For this review, use the dimensioned drawing (mm, ordinates from the lowest corner) and the shaded views. A direction names the side the tool comes from. Coordinates: 2 decimals unless noted, no trailing zeros. Order: outer loops, then holes, each group sorted by start corner. A loop starts at its lowest first (then second) coordinate and runs counter-clockwise, first axis right, second up. Notation, with made-up numbers: M -20.5,41 L 24.5,41 A25 ccw 24.5,69 Z; hole C 51.5,34 d4. An arc over 180 degrees is marked long. Use CSV: the item, a comma, the result in double quotes.
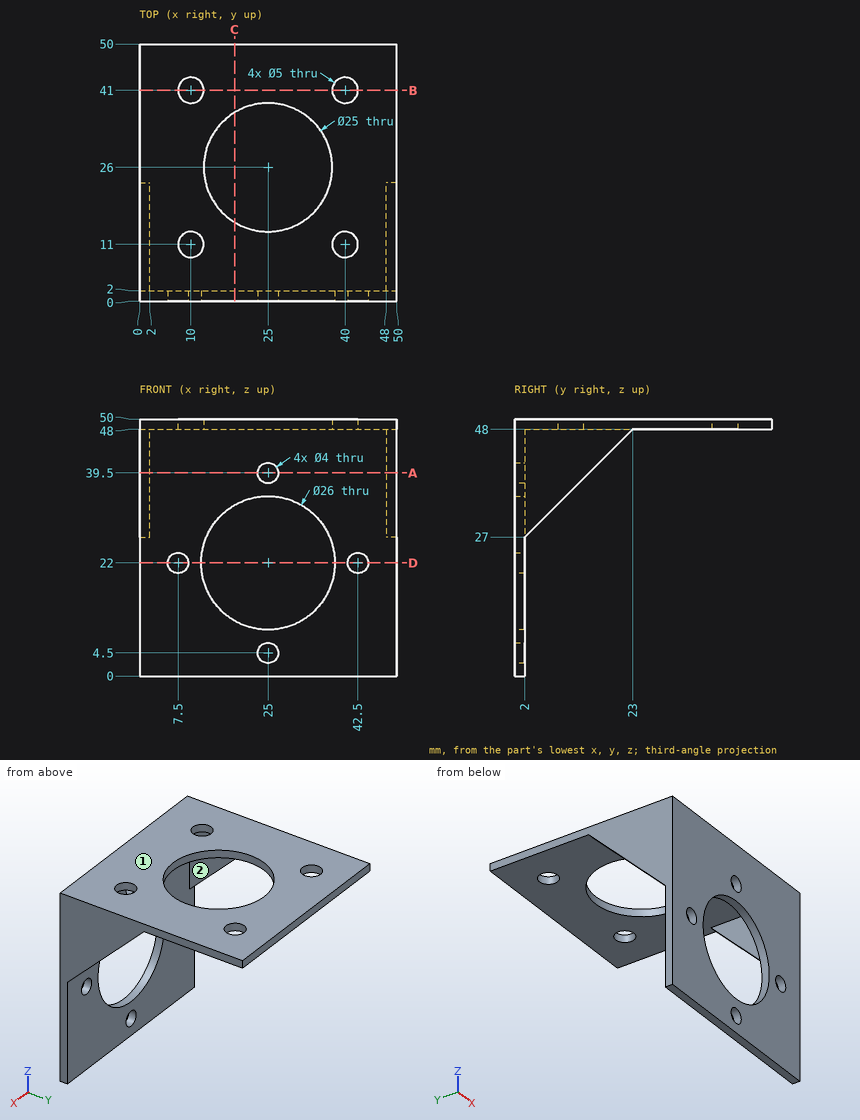
Item 1: Add section A-A on z = 39.5. State the section outline as (x, y) points.
Solutions:
outline,"M 0,0 L 23,0 L 23,2 L 2,2 L 2,14.5 L 0,14.5 Z; M 27,0 L 50,0 L 50,14.5 L 48,14.5 L 48,2 L 27,2 Z"
Item 2: To check wall thickness, follow line 1 along Y through (x, z) = (10, 48.6); line 2 along X through (y, z) = (7, 44); line 3 along X through (y, z) = (1, 4.5). State the ranges of each line that lie inside material, in increasing order. Write a range as [from, to].
Solutions:
line 1,"[0, 8.5], [13.5, 38.5], [43.5, 50]"
line 2,"[0, 2], [48, 50]"
line 3,"[0, 23], [27, 50]"
Item 3: Add section D-D on z = 22. State the section outline as (x, y) points, and give its area (3 significant figures).
Solutions:
outline,"M 0,0 L 5.5,0 L 5.5,2 L 0,2 Z; M 9.5,0 L 12,0 L 12,2 L 9.5,2 Z; M 38,0 L 40.5,0 L 40.5,2 L 38,2 Z; M 44.5,0 L 50,0 L 50,2 L 44.5,2 Z"
area,"32.0 mm^2"
Item 4: Clearance check with flat-ended pins moving along their axes: pin 1 Ø5 at (x, z) = (26, 34) entering from +Y; pin 2 Ø6 at (x, y) = (40, 41) entering from -Z; pin 3 Ø2 at (x, z) = (44, 13) entering from -Y; pin 4 Ø3.5 at (x, z) = (25, 4.5) entering from -Y. State where each tip first meets the part, or that it passes through.
Solutions:
pin 1,"y = 2"
pin 2,"z = 48"
pin 3,"y = 0"
pin 4,"through"
Item 5: For the marked faces 1 and 2, list the 3-axis set-ups (+Z, -Z, +X, -X, +Y, -Y) from which the entire face can be reached by the end or side of a thin tool; tool diameter is ignored.
Solutions:
face 1,"+Z, +X, -X, +Y, -Y"
face 2,"-Z, +Y"
Item 6: Add section B-B on y = 41. State the section outline as (x, z) points, and give its area (3 significant figures).
Solutions:
outline,"M 0,48 L 7.5,48 L 7.5,50 L 0,50 Z; M 12.5,48 L 37.5,48 L 37.5,50 L 12.5,50 Z; M 42.5,48 L 50,48 L 50,50 L 42.5,50 Z"
area,"80.0 mm^2"
Item 7: Add section C-C on x = 18.5. State the section outline as (y, z) points.
Solutions:
outline,"M 0,0 L 2,0 L 2,10.74 L 0,10.74 Z; M 0,33.26 L 2,33.26 L 2,48 L 15.32,48 L 15.32,50 L 0,50 Z; M 36.68,48 L 50,48 L 50,50 L 36.68,50 Z"
